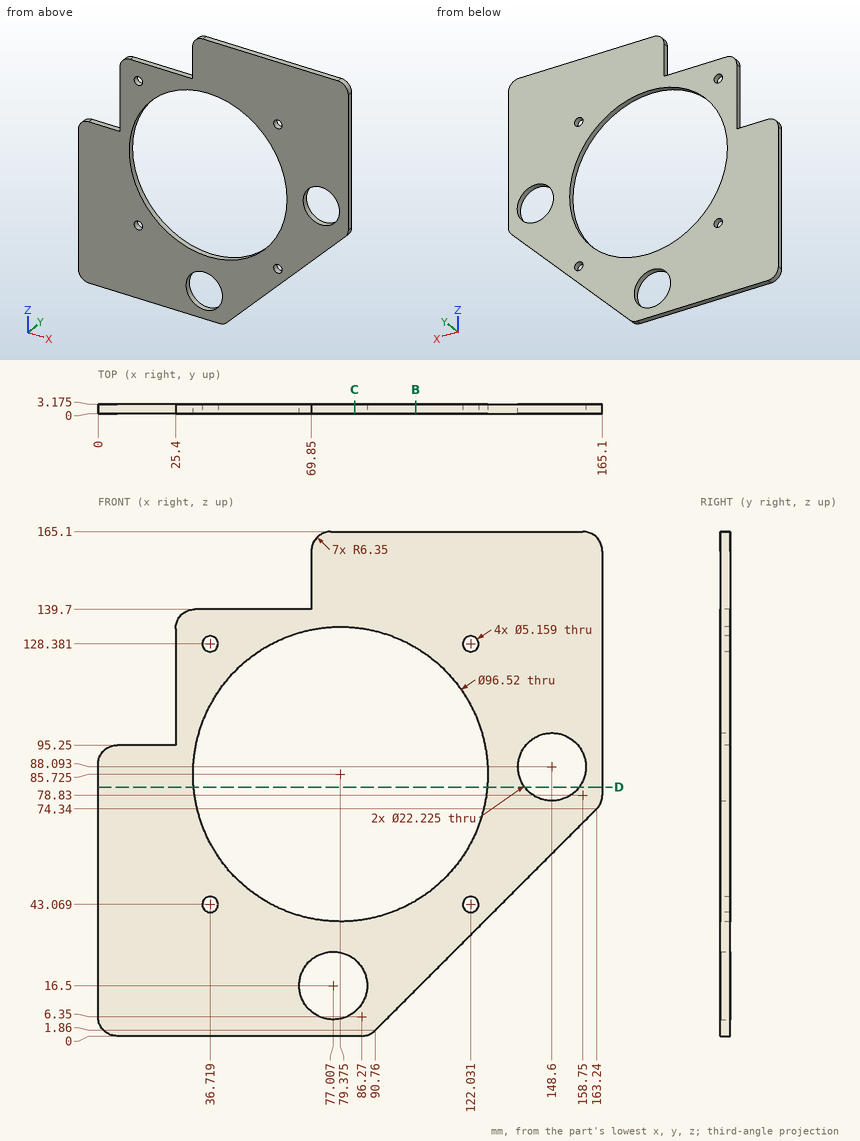
Source: three-view drawing plus pictorial views. Frame: mm from the lowest corner of the part. Coordinates: 2 decimals unless noted, no trailing zeros. Order: outer loops, then holes, each group sorted by start corner. A loop starts at its lowest first (then second) coordinate and runs counter-clockwise, first axis right, second up. Notation, with made-up numbers: M -26.75,39 L -20.75,39 A14 cw -20.75,59 Z; hole C -16,38 d9. An arc over 180 degrees is marked long. One line per question, with ' | ' between items.
Item 1: Section D-D (z = 81.5). Give the number of separate pieces and of enclosed holes in the cut face, then the cut area to 3 significant figures.
Geometry results:
separate pieces: 3 | enclosed holes: 0 | area: 162 mm^2
Item 2: Pin query (flat end, axial travel): pin 1 (1.6 mm diameter, centred on x = 45.5, y = 1.5, fed in from +Z); pin 2 (1 mm diameter, centred on y = 1.5, z = 106, fed in from -X); pin 3 (1.6 mm diameter, centred on x = 17, y = 1, fed in from +Z). Return the tip coordinate at first contact, or that it passes through.
Geometry results:
pin 1: stops at z = 139.7 | pin 2: stops at x = 25.4 | pin 3: stops at z = 95.25
Item 3: Ray query, line 1 along Z through (x, y) = (74, 1.6) (1 decimal); line 2 along Z through (x, y) = (80, 2.6); line 3 along X through (y, z) = (1.7, 129.5) (1 decimal). Return the intervals inside material, ascending.
Geometry results:
line 1: z = 0 to 5.8, 27.2 to 37.8, 133.7 to 164.7 | line 2: z = 0 to 5.8, 27.2 to 37.47, 133.98 to 165.1 | line 3: x = 25.4 to 34.4, 39 to 59.1, 99.7 to 119.7, 124.4 to 165.1
Item 4: Section C-C (x = 84). Output: boundary loops of the cut face in (y, z) (1 decimal).
Geometry results:
outline: M 0,0 L 3.2,0 L 3.2,7.9 L 0,7.9 Z; M 0,25.1 L 3.2,25.1 L 3.2,37.7 L 0,37.7 Z; M 0,133.8 L 3.2,133.8 L 3.2,165.1 L 0,165.1 Z
Item 5: Section B-B (x = 104). Output: boundary loops of the cut face in (y, z) (1 decimal), then the cut area to 3 significant figures.
Geometry results:
outline: M 0,15.1 L 3.2,15.1 L 3.2,44.2 L 0,44.2 Z; M 0,127.2 L 3.2,127.2 L 3.2,165.1 L 0,165.1 Z | area: 213 mm^2
